```python
from build123d import *

# Parameters (mm, degrees)
SKETCH1_W           = 48
SKETCH1_H           = 33
BOSS_EXTRUDE1_DEPTH = 1.7
SKETCH2_W           = 8
SKETCH2_H           = 21
BOSS_EXTRUDE2_DEPTH = 6
SKETCH3_R           = 1.5
CUT_EXTRUDE1_DEPTH  = 59.557663888
SKETCH4_W           = 36.5
SKETCH4_H           = 33
BOSS_EXTRUDE3_DEPTH = 1
SKETCH6_W           = 40
SKETCH6_H           = 17.6
BOSS_EXTRUDE4_DEPTH = 1.8


with BuildPart() as part:
    # Sketch1 → Boss-Extrude1 (new body)
    with BuildSketch(Plane(origin=(0, 0, 0), x_dir=(1, 0, 0), z_dir=(0, 1, 0))):
        with Locations((24, 16.5)):
            Rectangle(SKETCH1_W, SKETCH1_H)
    extrude(amount=BOSS_EXTRUDE1_DEPTH)

    # Sketch2 → Boss-Extrude2 (add)
    with BuildSketch(Plane(origin=(0, 1.7, 0), x_dir=(1, 0, 0), z_dir=(0, 1, 0))):
        with Locations((44, 16.5)):
            Rectangle(SKETCH2_W, SKETCH2_H)
    extrude(amount=BOSS_EXTRUDE2_DEPTH)

    # Sketch3 → Cut-Extrude1 (cut, through all)
    with BuildSketch(Plane(origin=(0, 1.7, 0), x_dir=(1, 0, 0), z_dir=(0, 1, 0))):
        with Locations(Location((2.5, 2.5, 0), (0, 0, 270))):
            Circle(SKETCH3_R)
        with Locations(Location((45.5, 2.5, 0), (0, 0, 90))):
            Circle(SKETCH3_R)
        with Locations(Location((45.5, 30.5, 0), (0, 0, 270))):
            Circle(SKETCH3_R)
        with Locations(Location((2.5, 30.5, 0), (0, 0, 90))):
            Circle(SKETCH3_R)
    extrude(amount=-CUT_EXTRUDE1_DEPTH, mode=Mode.SUBTRACT)

    # Sketch4 → Boss-Extrude3 (add)
    with BuildSketch(Plane(origin=(0, 0, 0), x_dir=(-1, 0, 0), z_dir=(0, -1, 0))):
        with Locations((-24, 16.5)):
            Rectangle(SKETCH4_W, SKETCH4_H)
    extrude(amount=BOSS_EXTRUDE3_DEPTH)

    # Sketch6 → Boss-Extrude4 (add)
    with BuildSketch(Plane(origin=(0, 1.7, 0), x_dir=(1, 0, 0), z_dir=(0, 1, 0))):
        with Locations((20, 16.5)):
            Rectangle(SKETCH6_W, SKETCH6_H)
    extrude(amount=BOSS_EXTRUDE4_DEPTH)


solid = part.part
```
Source: CAD feature listing. Evaluate the final solid. Frame: model axes, mm. A direction names the side the tool comes from. Give positions to 0.01 mm unless a question says otherwise; leave off trailing zeros. Loops run counter-clockwise (first coordinate to the right, second up) from the corner with the lowest first, then second, coordinate; pieces in that order, holes last. Notation, with made-up numbers: (-21.5, 15) -> (-13.5, 15) arc R16 ccw to (-13.5, 46) -> close; hole circle Ø10 at (78.5, 41). An arc over 180 degrees is marked (long way). Put each result on its own line as item: value. Start each with the question number.
1) Material intervals for probe 1 along X at (y, z) = (1.3, -2.5); probe 2 along Z at (x, y) = (46, 0.5); probe 3 along Y at (x, z) = (20, -3), sorted ascending.
2) Reachability of faces 5 (the face through (44, 5, -6)), 6 (the face through (45, 0, -17)), 7 (the face through (44, 5, -27)), 8 (the face through (3, 0, -17)), 9 (the face through (20, 3.5, -17)) from +Z, -Z, +X, -X, +Y, -Y: full face, straight path, thin tool, end or side. Return the list, or none.
3) Cut plane B-B (z = -30.5). Return loops of the section in (x, y), then the cut area to 3 significant figures.
4) Contact query for flat-ended pins moving along their axis: P1, Ø3, axis at x = 44, y = 6, coming from the -Z side; P2, Ø6.5, axis at x = 1.5, z = -20, coming from the -Y side; P3, Ø1.5, axis at x = 37, z = -24.5, coming from the +Y side; P4, Ø1, axis at y = 4, z = -3.5, coming from the +X side. Output: stop coordinate, or through.
5) Cut plane D-D (x = 14). Return loops of the section in (y, z), then the cut area to 3 significant figures.
6) Cut plane A-A (x = 45.5). Return loops of the section in (y, z), then the cut area to 3 significant figures.
7) Draft query along X for faces 1 (the face through (48, 3, -16)), 2 (the face through (24, 0, -33)), 3 (the face through (5.75, -0.5, -16.3)), 4 (the face through (2.43, 0.86, -29)). Return one class per face: released by +X, released by -X, zero draft, split by the parting line, or undercut.
8) Cut plane C-C (z = -14.5). Return loops of the section in (x, y).
Results are:
1. probe 1: x = 0 to 1, 4 to 44, 47 to 48
1. probe 2: z = -33 to -31.91, -29.09 to -3.91, -1.09 to 0
1. probe 3: y = -1 to 1.7
2. face 5: +Z, +X, -X, +Y
2. face 6: +Z, -Z, +X, -Y
2. face 7: -Z, +X, -X, +Y
2. face 8: +Z, -Z, -X, -Y
2. face 9: +Z, -Z, -X, +Y
3. outline: (0, 0) -> (1, 0) -> (1, 1.7) -> (0, 1.7) -> close; (4, 0) -> (5.75, 0) -> (5.75, -1) -> (42.25, -1) -> (42.25, 0) -> (44, 0) -> (44, 1.7) -> (4, 1.7) -> close; (47, 0) -> (48, 0) -> (48, 1.7) -> (47, 1.7) -> close
3. area: 108 mm2
4. P1: stops at z = -27
4. P2: stops at y = 0
4. P3: stops at y = 3.5
4. P4: passes through
5. outline: (-1, -33) -> (1.7, -33) -> (1.7, -25.3) -> (3.5, -25.3) -> (3.5, -7.7) -> (1.7, -7.7) -> (1.7, 0) -> (-1, 0) -> close
5. area: 121 mm2
6. outline: (0, -33) -> (1.7, -33) -> (1.7, -32) -> (0, -32) -> close; (0, -29) -> (1.7, -29) -> (1.7, -27) -> (7.7, -27) -> (7.7, -6) -> (1.7, -6) -> (1.7, -4) -> (0, -4) -> close; (0, -1) -> (1.7, -1) -> (1.7, 0) -> (0, 0) -> close
6. area: 172 mm2
7. face 1: released by +X
7. face 2: zero draft
7. face 3: released by -X
7. face 4: undercut
8. outline: (0, 0) -> (5.75, 0) -> (5.75, -1) -> (42.25, -1) -> (42.25, 0) -> (48, 0) -> (48, 7.7) -> (40, 7.7) -> (40, 3.5) -> (0, 3.5) -> close
